Print and shaded views of the part. All mm, measured from the part's lowest x, y and z. Coordinates: 2 decimals unless noted, no trailing zeros. Order: outer loops, then holes, each group sorted by start corner. A loop starts at its lowest first (then second) coordinate and runs counter-clockwise, first axis right, second up. Notation, with made-up numbers: M 42.5,-34 L 63.5,-34 A25 ccw 63.5,-10 Z; hole C 75.25,87 d5. An arc over 180 degrees is marked long. Return JSON: item names as keys, results as strings.
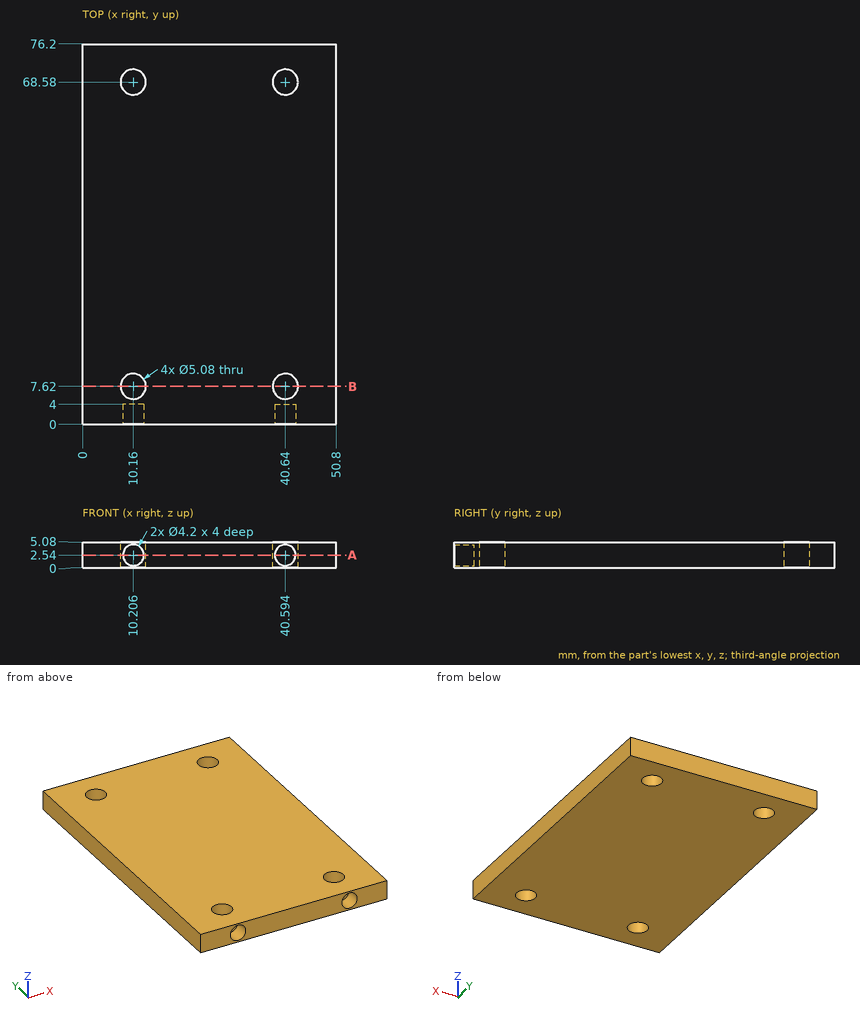
Item 1: Saw through at B-B (y = 7.62). Write the cut outline in (x, z).
Check result:
{"outline": "M 0,0 L 7.62,0 L 7.62,5.08 L 0,5.08 Z; M 12.7,0 L 38.1,0 L 38.1,5.08 L 12.7,5.08 Z; M 43.18,0 L 50.8,0 L 50.8,5.08 L 43.18,5.08 Z"}
Item 2: Saw through at A-A (z = 2.54). Write the cut outline in (x, y), and give its area (3 significant figures).
Check result:
{"outline": "M 0,0 L 8.11,0 L 8.11,4 L 12.31,4 L 12.31,0 L 38.49,0 L 38.49,4 L 42.69,4 L 42.69,0 L 50.8,0 L 50.8,76.2 L 0,76.2 Z; hole C 10.16,7.62 d5.08; hole C 10.16,68.58 d5.08; hole C 40.64,7.62 d5.08; hole C 40.64,68.58 d5.08", "area": "3,760 mm2"}
Item 3: Wall check: line 1 (X direction, y = 3.05, z = 2.54); line 2 (Y direction, x = 10.16, z = 3.8); line 3 (Y direction, x = 41, z = 1.5). Give the ranges that are in metal, low to high.
Check result:
{"line 1": "x = 0 to 8.11, 12.31 to 38.49, 42.69 to 50.8", "line 2": "y = 4 to 5.08, 10.16 to 66.04, 71.12 to 76.2", "line 3": "y = 4 to 5.11, 10.13 to 66.07, 71.09 to 76.2"}
Item 4: Drop a flat-ended pin along its axis: pin 1 Ø2.5 at (x, z) = (40.59, 2.54) entering from -Y. Give the stop position or say it passes through.
Check result:
{"pin 1": "stops at y = 4"}
